For this review, use the dimensioned drawing (mm, ordinates from the lowest corner) and the shaded views. A direction names the side the tool comes from. Coordinates: 2 decimals unless noted, no trailing zeros. Write each loop counter-clockwise with the first axis right and the second up, starting at its lowest first coordinate (ties: lowest second). Pieces come first, ordered by that corner, then holes. Notation, with made-up numbers: M 16,9 L 53,9 A30 cw 53,47 Z; hole C -12,44.25 d5. An arc over 180 degrees is marked long. One line per question, with ' | ' between items.
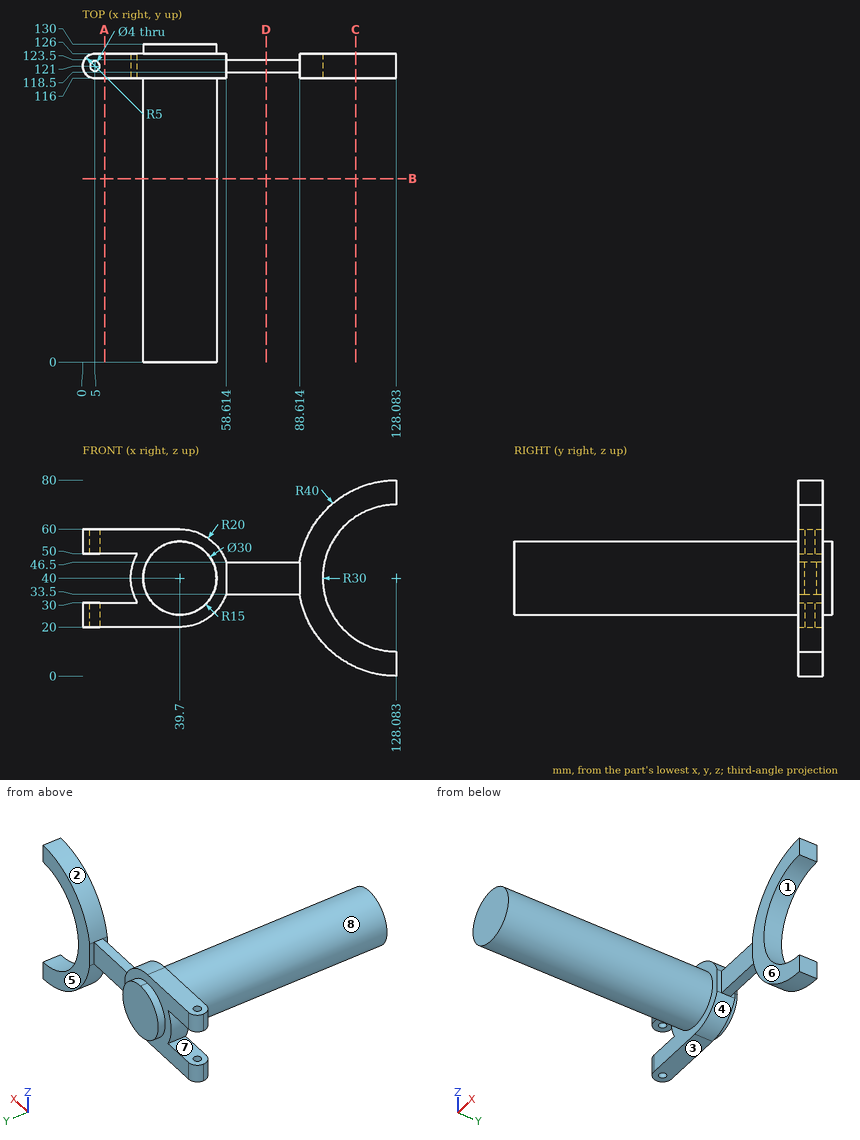
1) Insertion check: pin 1 Ø1.2 at (y, z) = (124.5, 41.5) entering from -X; pin 2 Ø8 at (x, y) = (9, 122) entering from -Z; pin 3 Ø14.5 at (x, z) = (68.5, 41.5) entering from +Y; pin 4 Ø5 at (y, z) = (94.5, 58) entering from +X. Each pin has a flat end and moves straight along its axis. Give the tip position at first contact, or say it passes through.
Responses:
pin 1: x = 19.72 | pin 2: z = 20 | pin 3: y = 123.5 | pin 4: through
2) The part is to be moulded in two halves that separate along X. For the marked faces 1, 2, 3 and 4, say which applies: +X half, -X half, draft (parallel to the pull), parting line (faces both ways), or undercut.
Responses:
face 1: +X half | face 2: undercut | face 3: draft | face 4: undercut
3) We need section B-B on y = 75. State the section outline as (x, z) points, then the cut area to 3 significant figures.
Responses:
outline: C 39.7,40 d30 | area: 707 mm^2
4) We need section D-D on x = 75. State the section outline as (y, z) points.
Responses:
outline: M 118.5,33.5 L 123.5,33.5 L 123.5,46.5 L 118.5,46.5 Z
5) We need section A-A on x = 9. State the section outline as (y, z) points, then the cut area to 3 significant figures.
Responses:
outline: M 116,20 L 126,20 L 126,30 L 116,30 Z; M 116,50 L 126,50 L 126,60 L 116,60 Z | area: 200 mm^2
6) We need section C-C on x = 111.5. State the section outline as (y, z) points.
Responses:
outline: M 116,3.6 L 126,3.6 L 126,15 L 116,15 Z; M 116,65 L 126,65 L 126,76.4 L 116,76.4 Z
7) To check wall thickness, follow line 1 along Y through (x, z) = (5, 24.5); line 2 along Z through (x, y) = (17, 118); line 3 along Z through (x, y) = (40.5, 36). State the ranges of each line that lie inside material, in increasing order. Write a range as [from, to].
Responses:
line 1: [116, 119], [123, 126] | line 2: [20, 30], [50, 60] | line 3: [25.02, 54.98]
8) Machinability: for the marked faces 5, 6, 7 and 8, which of the approach directions +Z, -Z, +X, -X, +Y, -Y give a long, thin tool a straight path to every point of the face, cutting with its end or side? Answer none if there is none.
Responses:
face 5: +Z, -Z, +X, +Y | face 6: +Z, -Z, +X, -Y | face 7: -X, +Y, -Y | face 8: -Y
